```python
from build123d import *

# Parameters (mm, degrees)
SKETCH1_R          = 12.7
BASE_FLANGE1_DEPTH = 1.5875
SKETCH12_R         = 2.413
CUT_EXTRUDE1_DEPTH = 53.579572138


# Sheet-metal steps are written as plain solids
with BuildPart() as part:
    # Sketch1 → Base-Flange1 (new body)
    with BuildSketch(Plane(origin=(0, 0, 0), x_dir=(1, 0, 0), z_dir=(0, 1, 0))):
        with BuildLine():
            Line((-22.225, 0), (-22.225, -47.625))
            Line((-22.225, -47.625), (22.225, -47.625))
            Line((22.225, -47.625), (22.225, 0))
            ThreePointArc((22.225, 0), (0, 22.225), (-22.225, 0))
        make_face()
        with Locations(Location((0, -9.525, 0), (0, 0, 270))):
            Circle(SKETCH1_R, mode=Mode.SUBTRACT)
    extrude(amount=-BASE_FLANGE1_DEPTH)

    # Sketch12 → Cut-Extrude1 (cut, through all)
    with BuildSketch(Plane.XZ.offset(1.5875)):
        with Locations(Location((15.875, 41.275, 0), (0, 0, 270))):
            Circle(SKETCH12_R)
        with Locations(Location((0, 41.275, 0), (0, 0, 270))):
            Circle(SKETCH12_R)
        with Locations(Location((-15.875, 41.275, 0), (0, 0, 270))):
            Circle(SKETCH12_R)
    extrude(amount=-CUT_EXTRUDE1_DEPTH, mode=Mode.SUBTRACT)


solid = part.part
```
Design review of the part built by this model. Coordinates are the model's own, in mm. Give positions to 0.01 mm unless a question says otherwise; leave off trailing zeros. Write each loop counter-clockwise with the first axis right and the second up, starting at its lowest first coordinate (ties: lowest second). Pieces come first, ordered by that corner, then holes.
(1) Mouldability with a two-part tool opening along X and no side actions: class faces 1 (the face through (10, 0, 20)), 2 (the face through (14.951, -0.805, 39.046)), 3 (the face through (-22.225, -1, 23)) as +X half, -X half, draft (parallel to the pull), parting line (faces both ways), or undercut.
Checked values:
face 1: draft
face 2: undercut
face 3: -X half
(2) Wall thickness on line 1 along X through (y, z) = (-0.1, 40) (3 decimals); line 2 along Z through (x, y) = (7, -0.8) (3 decimals); line 3 along X through (y, z) = (-0.9, 6.5) (3 decimals): over which ranges is each line inside the solid? List them lowest first.
Checked values:
line 1: x = -22.225 to -17.924, -13.826 to -2.049, 2.049 to 13.826, 17.924 to 22.225
line 2: z = -21.094 to -1.072, 20.122 to 47.625
line 3: x = -22.225 to -12.334, 12.334 to 22.225
(3) Add section C-C (x = 6.5). Give the boundary of the cut face in (y, z) (1 decimal).
Checked values:
outline: (-1.6, -21.3) - (0, -21.3) - (0, -1.4) - (-1.6, -1.4) - close; (-1.6, 20.4) - (0, 20.4) - (0, 47.6) - (-1.6, 47.6) - close
(4) Add section A-A (x = 0). Give the boundary of the cut face in (y, z) (1 decimal), and give its area (3 significant figures).
Checked values:
outline: (-1.6, -22.2) - (0, -22.2) - (0, -3.2) - (-1.6, -3.2) - close; (-1.6, 22.2) - (0, 22.2) - (0, 38.9) - (-1.6, 38.9) - close; (-1.6, 43.7) - (0, 43.7) - (0, 47.6) - (-1.6, 47.6) - close
area: 62.9 mm2
(5) Add section B-B (z = 19). Give the boundary of the cut face in (x, y) (1 decimal).
Checked values:
outline: (-22.2, -1.6) - (-8.5, -1.6) - (-8.5, 0) - (-22.2, 0) - close; (8.5, -1.6) - (22.2, -1.6) - (22.2, 0) - (8.5, 0) - close
(6) Add section D-D (y = -0.55). Give the boundary of the cut face in (x, z) (3 decimals), and give its area (3 significant figures).
Checked values:
outline: (-22.225, 0) arc R22.225 ccw to (22.225, 0) - (22.225, 47.625) - (-22.225, 47.625) - close; hole circle Ø4.826 at (-15.875, 41.275); hole circle Ø25.4 at (0, 9.525); hole circle Ø4.826 at (0, 41.275); hole circle Ø4.826 at (15.875, 41.275)
area: 2,330 mm2
